The drawing under review shows one solid part. Ordinate dimensions are in mm from its lowest x, y, z. A direction names the side the tool comes from. Give positions to 0.01 mm unless a question says otherwise; leave off trailing zeros. Write each loop counter-clockwise with the first axis right and the second up, starting at its lowest first coordinate (ties: lowest second). Pieces come first, ordered by that corner, then holes. Notation, with made-up numbers: (-26, 28.25) -> (20, 28.25) arc R22 ccw to (20, 60.25) -> close; hole circle Ø10 at (78.5, 31.5). An arc over 180 degrees is marked (long way). Use CSV: the item, a comma, the result in double quotes.
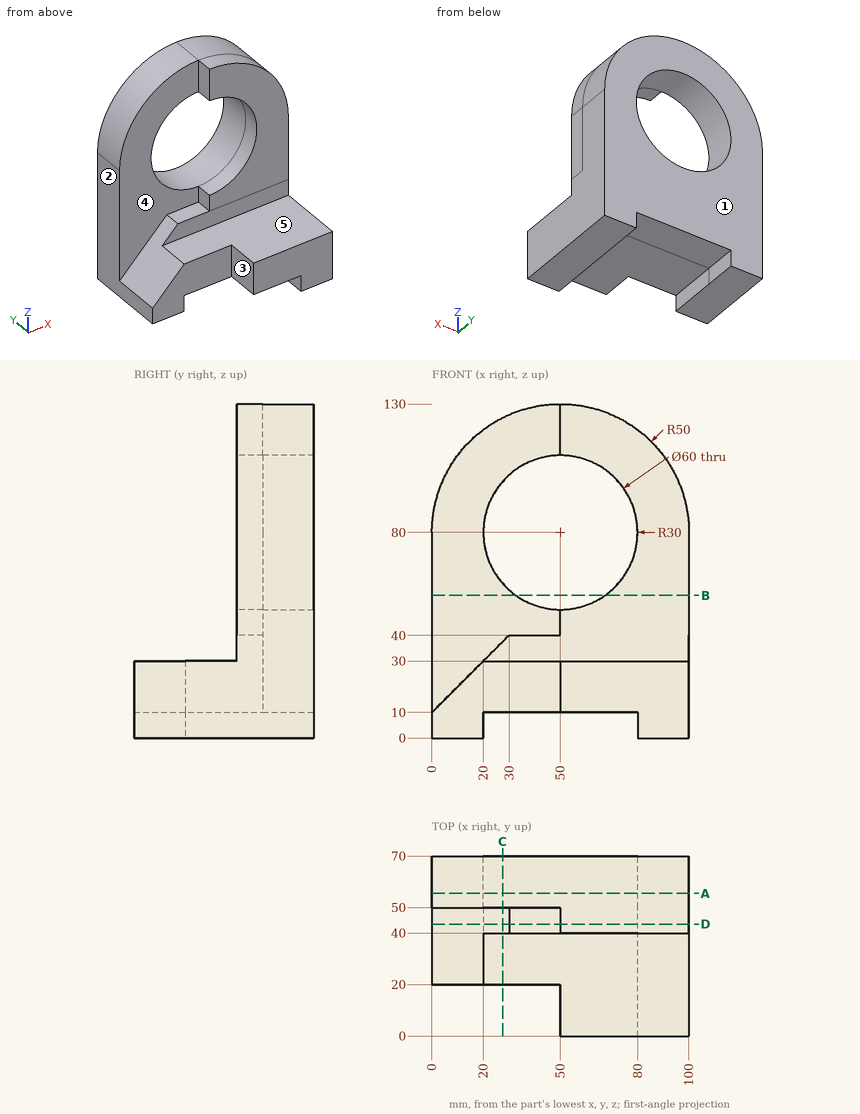
(1) Take a section at B-B (z = 55.5). Write out the cut boundary in (x, y).
Established:
outline,"(0, 50) -> (32.69, 50) -> (32.69, 70) -> (0, 70) -> close; (67.31, 40) -> (100, 40) -> (100, 70) -> (67.31, 70) -> close"
(2) Take a section at D-D (y = 43.5). Write out the cut boundary in (x, z), then the cut area to 3 significant figures.
Established:
outline,"(0, 0) -> (20, 0) -> (20, 10) -> (80, 10) -> (80, 0) -> (100, 0) -> (100, 80) arc R50 ccw to (50, 130) -> (50, 110) arc R30 cw to (50, 50) -> (50, 40) -> (30, 40) -> (0, 10) -> close"
area,"5,500 mm2"
(3) Clearance check with flat-ended pins moving along their axes: pin 1 (3 mm diameter, centred on y = 45, z = 55.5, fed in from -X); pin 2 (2 mm diameter, centred on x = 52, y = 43.5, fed in from -Z); pin 3 (5 mm diameter, centred on y = 14.5, z = 4, fed in from -X); pin 4 (10 mm diameter, centred on x = 74, z = 75, fed in from -Y). State where each tip first meets the part, or that it passes through.
Established:
pin 1,"stops at x = 64.97"
pin 2,"stops at z = 10"
pin 3,"stops at x = 80"
pin 4,"passes through"
(4) Take a section at C-C (x = 27.5). Write out the cut boundary in (y, z), then the cut area to 3 significant figures.
Established:
outline,"(20, 10) -> (70, 10) -> (70, 60.16) -> (50, 60.16) -> (50, 37.5) -> (40, 37.5) -> (40, 30) -> (20, 30) -> close; (50, 99.84) -> (70, 99.84) -> (70, 124.65) -> (50, 124.65) -> close"
area,"2,170 mm2"
(5) Tool access review of the marked faces 1, 2, 3, 4 and 5: name each direction out of +Z, -Z, +X, -X, +Y, -Y from which nothing blocks a thin tool from reaching the whole face with its end or side.
Established:
face 1,"+Z, -Z, +X, -X, +Y"
face 2,"+Z, -Z, -X, +Y, -Y"
face 3,"+Z, -Z, -X, -Y"
face 4,"+Z, -X, -Y"
face 5,"+Z, +X, -X, -Y"
(6) For line 1 along X through (y, z) = (58.75, 80); line 2 along Z through (x, y) = (50, 61.5); line 3 along Y through (x, z) = (35, 120.5), list the stretches that pass through material, from the lowest coordinate up. Write a range as [from, to].
Established:
line 1,"x = [0, 20], [80, 100]"
line 2,"z = [10, 50], [110, 130]"
line 3,"y = [50, 70]"
(7) Take a section at A-A (y = 55.5). Write out the cut boundary in (x, z).
Established:
outline,"(0, 0) -> (20, 0) -> (20, 10) -> (80, 10) -> (80, 0) -> (100, 0) -> (100, 80) arc R50 ccw to (0, 80) -> close; hole circle Ø60 at (50, 80)"
